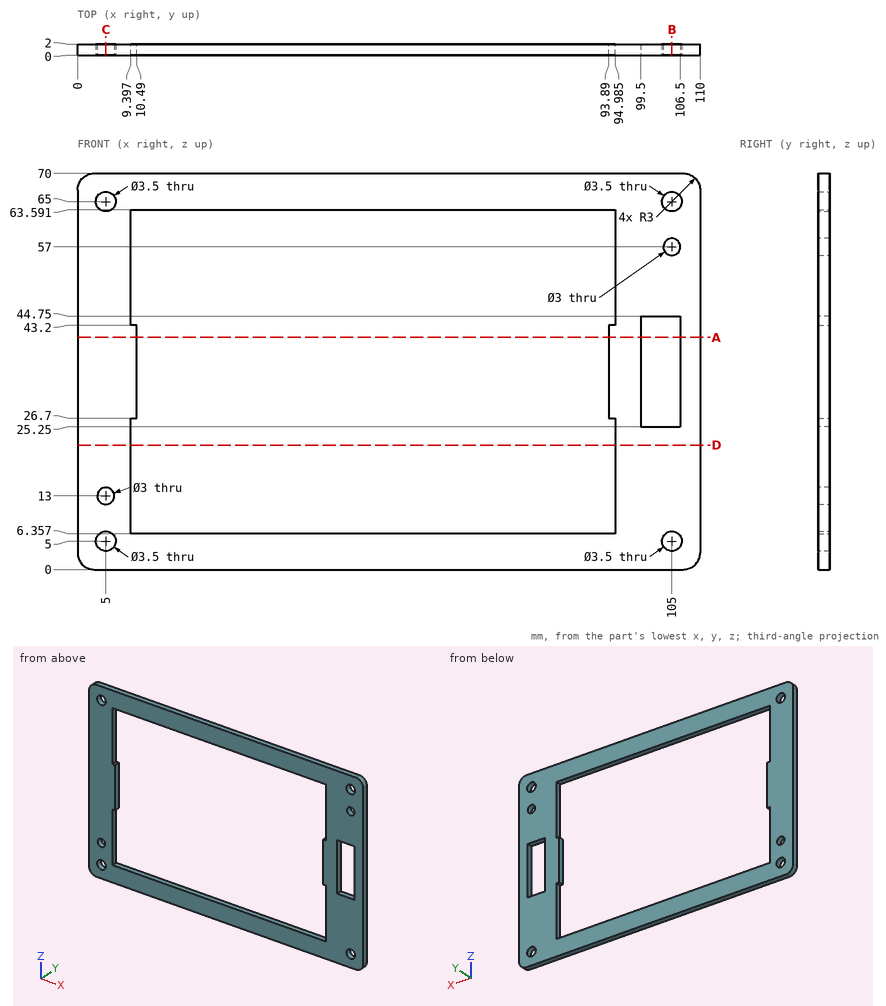
Study the drawing (mm; zero at the part's minimum x, y, z) and answer. Round coordinates to 2 decimals unless told otherwise and drop trailing zeros. Write each loop counter-clockwise with the first axis right and the second up, starting at its lowest first coordinate (ties: lowest second). Pieces come first, ordered by that corner, then holes. Notation, with made-up numbers: (83, -22.75) - (107, -22.75) arc R10 ccw to (107, -15.75) - close; hole circle Ø7 at (-6.75, -20.75). An arc over 180 degrees is marked (long way). Use a Markdown table: item, result. Add a question column.
1. Consider line 1 (Z direction, x = 105, y = 1.15); line 2 (X direction, y = 0.7, z = 13) (1 decimal); line 3 (X direction, y = 0.9, z = 37.5). Determine where each line is inside the solid, lowest interval first.
2. A flat-ended cylindrical pin translates along its axis: P1, Ø10, axis at x = 89, z = 16.5, coming from the +Y side. Find the tip coordinate at first contact, or state that the pin passes through.
3. The part is cut by section A-A (z = 41). Write down the section's boundary in (x, y).
4. The part is cut by section D-D (z = 22). Write down the section's boundary in (x, y) (1 decimal).
5. The part is cut by section B-B (x = 105). Write down the section's boundary in (y, z).
6. The part is cut by section C-C (x = 5). Write down the section's boundary in (y, z), and give its area (3 significant figures).
Reported:
| question | item | result |
|---|---|---|
| 1 | line 1 | 0 to 3.25, 6.75 to 25.25, 44.75 to 55.5, 58.5 to 63.25, 66.75 to 70 |
| 1 | line 2 | 0 to 3.5, 6.5 to 9.4, 95 to 110 |
| 1 | line 3 | 0 to 10.49, 93.89 to 99.5, 106.5 to 110 |
| 2 | P1 | through |
| 3 | outline | (0, 0) - (10.49, 0) - (10.49, 2) - (0, 2) - close; (93.89, 0) - (99.5, 0) - (99.5, 2) - (93.89, 2) - close; (106.5, 0) - (110, 0) - (110, 2) - (106.5, 2) - close |
| 4 | outline | (0, 0) - (9.4, 0) - (9.4, 2) - (0, 2) - close; (95, 0) - (110, 0) - (110, 2) - (95, 2) - close |
| 5 | outline | (0, 0) - (2, 0) - (2, 3.25) - (0, 3.25) - close; (0, 6.75) - (2, 6.75) - (2, 25.25) - (0, 25.25) - close; (0, 44.75) - (2, 44.75) - (2, 55.5) - (0, 55.5) - close; (0, 58.5) - (2, 58.5) - (2, 63.25) - (0, 63.25) - close; (0, 66.75) - (2, 66.75) - (2, 70) - (0, 70) - close |
| 6 | outline | (0, 0) - (2, 0) - (2, 3.25) - (0, 3.25) - close; (0, 6.75) - (2, 6.75) - (2, 11.5) - (0, 11.5) - close; (0, 14.5) - (2, 14.5) - (2, 63.25) - (0, 63.25) - close; (0, 66.75) - (2, 66.75) - (2, 70) - (0, 70) - close |
| 6 | area | 120 mm^2 |
